from build123d import *

# Parameters (mm, degrees)
F1_DEPTH  = 5
F4_DEPTH  = 5
F7_DEPTH  = 5.42
F11_DEPTH = 2
F14_DEPTH = 2
F8_W      = 30
F8_H      = 95.5248658727
F15_DEPTH = 2
F17_DEPTH = 102.5
F18_DEPTH = 2
F19_DEPTH = 239
F22_DEPTH = 2
F25_DEPTH = 25
F27_W     = 101.7516627908
F27_H     = 74.3317976594
F28_DEPTH = 25
F30_W     = 3.562554135
F30_H     = 2.8552263975
F31_DEPTH = 25
F33_W     = 167.9849326611
F33_H     = 135.5820912868
F34_DEPTH = 25
F35_DEPTH = 25
F36_DEPTH = 5
F37_DEPTH = 5
F6_W      = 160
F6_H      = 95.5248658727
F38_DEPTH = 5
F39_R     = 1.7
F40_DEPTH = 9.9
F41_DEPTH = 20
F42_R     = 1.7
F43_DEPTH = 25
F44_R     = 5.3
F45_DEPTH = 5
F46_R     = 5.3
F47_DEPTH = 5
F48_DEPTH = 154
F49_DEPTH = 5
F50_DEPTH = 5


with BuildPart() as f1:
    # F0 (on Front) → F1 (new body)
    with BuildSketch(Plane.XZ):
        Polygon((-300, 20), (-300, 0), (0, 0), (0, 175), (-30, 175), (-30, 95), (-70, 95), (-75, 90), (-75, 85), (-140, 20), align=None)
    extrude(amount=F1_DEPTH)

    # F3 (on offset) → F4 (join)
    with BuildSketch(Plane(origin=(0, 0, 85), x_dir=(1, 0, 0), z_dir=(0, 0, -1))):
        Polygon((0, -157.818160031), (0, 0), (-70, 0), (-140, -70), (-300, -70), (-300, -157.818160031), align=None)
    extrude(amount=-F4_DEPTH)



with BuildPart() as f7:
    # F0 (on Front) → F7 (new body)
    with BuildSketch(Plane.XZ):
        Polygon((-300, 20), (-300, 0), (0, 0), (0, 175), (-30, 175), (-30, 95), (-70, 95), (-75, 90), (-75, 85), (-140, 20), align=None)
    extrude(amount=F7_DEPTH)


with BuildPart() as f1_1:
    add(f1.part)

    add(f7.part)  # F11 merges F7
    # F10 (on 3pt) → F11 (join)
    with BuildSketch(Plane(origin=(-55.9001782531, -51.9073083779, 55.9001782531), x_dir=(-0.3881029321, 0.8359140076, 0.3881029321), z_dir=(0.5910804633, 0.5488604302, -0.5910804633))):
        Polygon((62.0964691388, -84.8528137424), (145.837140261, -38.8908729653), (62.0964691388, 7.0710678119), align=None)
    extrude(amount=F11_DEPTH)


with BuildPart() as f14:
    # F13 (on 3pt) → F14 (new body)
    with BuildSketch(Plane.XY.offset(85)):
        Polygon((-75, 0), (-70, 0), (-140, 70), align=None)
    extrude(amount=-F14_DEPTH)


with BuildPart() as f15:
    # F8 (on 3pt) → F15 (new body)
    with BuildSketch(Plane(origin=(0, -9.9726027397, 10.7397260274), x_dir=(1, 0, 0), z_dir=(0, 0.6804510994, -0.7327934916))):
        with Locations((-125, -61.3714549237)):
            Rectangle(F8_W, F8_H)
    extrude(amount=-F15_DEPTH)


with BuildPart() as f17_tool:
    # F17 (cut): a face of the model
    f17_faces = [f1_1.part.faces().sort_by_distance(p)[0] for p in [
        (-129.156432847, 97.5448991734, 85),
    ]]
    extrude(f17_faces, amount=-F17_DEPTH)


with BuildPart() as f1_2:
    add(f1_1.part)

    # F17: cut by f17_tool
    add(f17_tool.part, mode=Mode.SUBTRACT)


    add(f14.part)  # F18 merges F14


with BuildPart() as f15_1:
    add(f15.part)

    # F17: cut by f17_tool
    add(f17_tool.part, mode=Mode.SUBTRACT)


with BuildPart() as f1_3:
    add(f1_2.part)

    add(f15_1.part)  # F18 merges F15
    # F16 (on face) → F18 (join)
    with BuildSketch(Plane.XZ):
        Polygon((-45, 85), (-75, 85), (-140, 20), (-110, 20), align=None)
    extrude(amount=-F18_DEPTH)

    # F0 (on Front) → F19 (cut)
    with BuildSketch(Plane.XZ):
        Polygon((-300, 20), (-300, 0), (0, 0), (0, 175), (-30, 175), (-30, 95), (-70, 95), (-75, 90), (-75, 85), (-140, 20), align=None)
    extrude(amount=F19_DEPTH, mode=Mode.SUBTRACT)

    # F21 (on 3pt) → F22 (join)
    with BuildSketch(Plane(origin=(0, 0, 85), x_dir=(1, 0, 0), z_dir=(0, 0, -1))):
        Polygon((-110, -70), (-45, 0), (-75, 0), (-140, -70), align=None)
    extrude(amount=F22_DEPTH)

    # F24 (on 3pt) → F25 (cut)
    with BuildSketch(Plane(origin=(0, -9.9726027397, 10.7397260274), x_dir=(1, 0, 0), z_dir=(0, -0.6804510994, 0.7327934916))):
        Polygon((-152.044788003, 115.9684211016), (-152.044788003, 9.7816493362), (-52.4809733033, 8.1501184031), (-52.4809733033, 115.9684211016), align=None)
    extrude(amount=-F25_DEPTH, mode=Mode.SUBTRACT)

    # F27 (on 3pt) → F28 (cut)
    with BuildSketch(Plane(origin=(-55.9001782531, -51.9073083779, 55.9001782531), x_dir=(-0.3881029321, 0.8359140076, 0.3881029321), z_dir=(0.5910804633, 0.5488604302, -0.5910804633))):
        with Locations((109.982162714, -56.3623122871)):
            Rectangle(F27_W, F27_H)
    extrude(amount=-F28_DEPTH, mode=Mode.SUBTRACT)

    # F30 (on 3pt) → F31 (cut)
    with BuildSketch(Plane(origin=(-52.6598984772, 0, 3.7614213198), x_dir=(0, 1, 0), z_dir=(0.9974586998, 0, -0.07124705))):
        with Locations((1.0092993034, 80.4627463222)):
            Rectangle(F30_W, F30_H)
    extrude(amount=F31_DEPTH, mode=Mode.SUBTRACT)

    # F33 (on 3pt) → F34 (cut)
    with BuildSketch(Plane(origin=(-46.9394598514, -42.3413086823, 45.598332427), x_dir=(0.3896444557, -0.8395868317, -0.378511757), z_dir=(-0.6022183228, -0.5432255075, 0.585012085))):
        with Locations((-70.4560130835, -7.8508025035)):
            Rectangle(F33_W, F33_H)
    extrude(amount=-F34_DEPTH, mode=Mode.SUBTRACT)

    # F35 (cut): a face of the model
    f35_faces = [f1_3.faces().sort_by_distance(p)[0] for p in [
        (-138.1104971586, 68.1104971586, 85.064982902),
    ]]
    extrude(f35_faces, amount=-F35_DEPTH, mode=Mode.SUBTRACT)

    # F3 (on offset) → F36 (join)
    with BuildSketch(Plane(origin=(0, 0, 85), x_dir=(1, 0, 0), z_dir=(0, 0, -1))):
        Polygon((0, -157.818160031), (0, 0), (-70, 0), (-140, -70), (-300, -70), (-300, -157.818160031), align=None)
    extrude(amount=-F36_DEPTH)

    # F0 (on Front) → F37 (join)
    with BuildSketch(Plane.XZ):
        Polygon((-300, 20), (-300, 0), (0, 0), (0, 175), (-30, 175), (-30, 95), (-70, 95), (-75, 90), (-75, 85), (-140, 20), align=None)
    extrude(amount=F37_DEPTH)

    # F39 (on face) → F40 (cut)
    with BuildSketch(Plane.XZ.offset(5)):
        with Locations((-115.7, 34.7)):
            Circle(F39_R)
        with Locations((-84.7, 65.7)):
            Circle(F39_R)
    extrude(amount=-F40_DEPTH, mode=Mode.SUBTRACT)

    # F41 (cut): a face of the model
    f41_faces = [f1_3.faces().sort_by_distance(p)[0] for p in [
        (-110, 34.1938617489, 53.1056998046),
    ]]
    extrude(f41_faces, amount=-F41_DEPTH, mode=Mode.SUBTRACT)

    # F42 (on face) → F43 (cut)
    with BuildSketch(Plane.XY.offset(90)):
        with Locations((-86.2, 30.7)):
            Circle(F42_R)
        with Locations((-115.7, 59.7)):
            Circle(F42_R)
    extrude(amount=-F43_DEPTH, mode=Mode.SUBTRACT)

    # F44 (on face) → F45 (join)
    with BuildSketch(Plane(origin=(0, 2, 0), x_dir=(-1, 0, 0), z_dir=(0, 1, 0))):
        with Locations((115.7, 34.7)):
            Circle(F44_R)
        Polygon((118.9331615075, 34.7), (117.3165807537, 31.9), (114.0834192463, 31.9), (112.4668384925, 34.7), (114.0834192463, 37.5), (117.3165807537, 37.5), align=None, mode=Mode.SUBTRACT)
        with Locations((84.7, 65.7)):
            Circle(F44_R)
        Polygon((87.9331615075, 65.7), (86.3165807537, 62.9), (83.0834192463, 62.9), (81.4668384925, 65.7), (83.0834192463, 68.5), (86.3165807537, 68.5), align=None, mode=Mode.SUBTRACT)
    extrude(amount=F45_DEPTH)

    # F46 (on face) → F47 (join)
    with BuildSketch(Plane(origin=(0, 0, 83), x_dir=(1, 0, 0), z_dir=(0, 0, -1))):
        with Locations((-115.7, -59.7)):
            Circle(F46_R)
        Polygon((-112.4668384925, -59.7), (-114.0834192463, -62.5), (-117.3165807537, -62.5), (-118.9331615075, -59.7), (-117.3165807537, -56.9), (-114.0834192463, -56.9), align=None, mode=Mode.SUBTRACT)
        with Locations((-86.2, -30.7)):
            Circle(F46_R)
        Polygon((-82.9668384925, -30.7), (-84.5834192463, -33.5), (-87.8165807537, -33.5), (-89.4331615075, -30.7), (-87.8165807537, -27.9), (-84.5834192463, -27.9), align=None, mode=Mode.SUBTRACT)
    extrude(amount=F47_DEPTH)

    # F39 (on face) → F49 (cut)
    with BuildSketch(Plane.XZ.offset(5)):
        Polygon((-140, 20), (-300, 20), (-300, 0), (0, 0), (0, 175), (-30, 175), (-30, 95), (-70, 95), (-75, 90), (-75, 85), align=None)
        with Locations((-115.7, 34.7)):
            Circle(F39_R, mode=Mode.SUBTRACT)
        with Locations((-84.7, 65.7)):
            Circle(F39_R, mode=Mode.SUBTRACT)
    extrude(amount=-F49_DEPTH, mode=Mode.SUBTRACT)

    # F42 (on face) → F50 (cut)
    with BuildSketch(Plane.XY.offset(90)):
        Polygon((0, 0), (0, 157.818160031), (-300, 157.818160031), (-300, 70), (-140, 70), (-70, 0), align=None)
        with Locations((-86.2, 30.7)):
            Circle(F42_R, mode=Mode.SUBTRACT)
        with Locations((-115.7, 59.7)):
            Circle(F42_R, mode=Mode.SUBTRACT)
    extrude(amount=-F50_DEPTH, mode=Mode.SUBTRACT)


with BuildPart() as f38:
    # F6 (on 3pt) → F38 (new body)
    with BuildSketch(Plane(origin=(0, -9.9726027397, 10.7397260274), x_dir=(1, 0, 0), z_dir=(0, 0.6804510994, -0.7327934916))):
        with Locations((-220, -61.3714549237)):
            Rectangle(F6_W, F6_H)
    extrude(amount=F38_DEPTH)

    # F6 (on 3pt) → F48 (cut)
    with BuildSketch(Plane(origin=(0, -9.9726027397, 10.7397260274), x_dir=(1, 0, 0), z_dir=(0, 0.6804510994, -0.7327934916))):
        with Locations((-220, -61.3714549237)):
            Rectangle(F6_W, F6_H)
    extrude(amount=F48_DEPTH, mode=Mode.SUBTRACT)


solid = f1_3.part
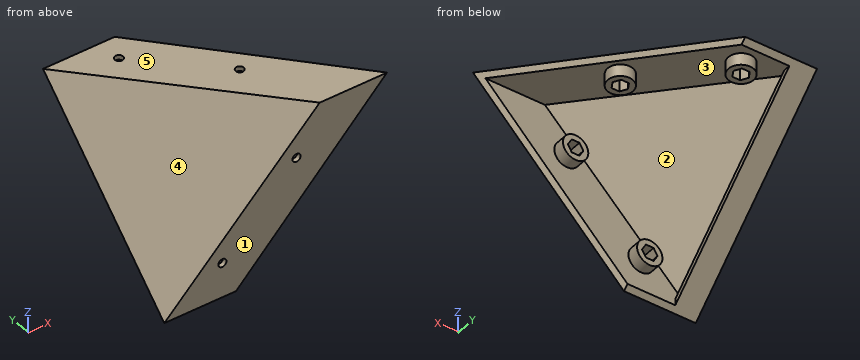
Verification items for the finished model (mm, model axes). Face numbers are marked on the shaded views. A direction names the side the tool comes from. Give positions to 0.01 mm unless a question says otherwise; leave off trailing zeros. Loops run counter-clockwise (first coordinate to the right, second up) from the corner with the lowest first, then second, coordinate; pieces in that order, holes last.
1. Cross-section at B-B on x = -78. Record the cut outline in (y, z).
Derived:
outline: (0, 52.94) - (2, 54.8) - (2, 80.47) - (4.72, 83) - (32.37, 83) - (34.52, 85) - (3.23, 85) - (0, 82) - close
2. Tool access check on the marked faces 1 and 2. Record the directions out of +Z, -Z, +X, -X, +Y, -Y that give a thin tool (end or side, any length) a straight path to the whole face; none if there is none.
Derived:
face 1: +Z, -Z, +X, -X, -Y
face 2: none
3. Material ranges on probe 1 along X at (y, z) = (6.5, 67); probe 2 along Y at (x, z) = (-91, 43); probe 3 along Y at (x, z) = (-115, 84), recorded low to high.
Derived:
probe 1: x = -99.04 to -95.65, -89.84 to -87.18, -82.22 to -79.56
probe 2: y = 0 to 2
probe 3: y = 42 to 58.15, 61.25 to 68.92
4. Release check for a two-part mould opening along X. For the marked faces 3, 4 and 5 record: +X half, -X half, draft (parallel to the pull), parting line (faces both ways), or undercut.
Derived:
face 3: undercut
face 4: -X half
face 5: draft
5. Go/stop test with flat-tipped pins: P1, Ø1, axis at y = 31, z = 72, coming from the -X side; P2, Ø3.5, axis at x = -115.5, y = 5.5, coming from the +Z side; P3, Ø2.5, axis at x = -115.5, z = 81.5, coming from the +Y side. Record where each tip stops, or that it passes through.
Derived:
P1: stops at x = -117.47
P2: stops at z = 52
P3: stops at y = 65
6. Cross-section at A-A on z = 44. Record the cut outline in (x, y), and give its area (3 significant figures).
Derived:
outline: (-140, 25.85) - (-116, 0) - (-86.69, 0) - (-88.49, 2) - (-114.47, 2) - (-133.89, 22.91) - (-130, 22.91) - (-130, 25.85) - close
area: 155 mm2
